Verification items for this drawing (mm, ordinates from the low corner). A direction names the side the tool comes from. Give positions to 0.01 mm unless a question says otherwise; leave off trailing zeros. Loops run counter-clockwise (first coordinate to the right, second up) from the corner with the lowest first, then second, coordinate; pieces in that order, holes last. Notation, with made-up numbers: (-0.5, -25) -> (32.5, -25) arc R17 cw to (32.5, -11) -> close; hole circle Ø5 at (-11, 57). An arc over 180 degrees is marked (long way). Write each question's results on one line, items separated by ' | '. Start each with the question number.
Item 1: Cross-section at B-B on z = 60. Enter the section's corners in (x, y), then the cut area to 3 significant figures.
Item 2: Cross-section at D-D on x = 20. Enter the section's corners in (y, z) (1 decimal).
Item 3: Scan lines: line 1 along Z through (x, y) = (24.5, 15); line 2 along Z through (x, y) = (39, 15); line 3 along Y through (x, z) = (63.5, 15). Record each from-to range of solid material in increasing order.
Item 4: Access from +Z, -Z, +X, -X, +Y, -Y to the whole of each face (thin tool, end or side, straight path). Record for the marked faces 5, 6, 7, 8 and 9.
Item 5: Cross-section at A-A on x = 41. Enter the section's corners in (y, z) (1 decimal).
Item 6: Cross-section at C-C on z = 77. Enter the section's corners in (x, y).
Item 7: Mould release check, pull along Z, two halves, no side actions. Record for the marked faces 1, 2, 3 and 4: pulls with the +Z half, pulls with the -Z half, needs draft (parallel to the pull), parting line crosses it, or undercut.
Item 8: Gauge pin test, flat ends, axial feed: pin 1 Ø15 at (y, z) = (11, 54) entering from -X; pin 2 Ø15 at (y, z) = (15.5, 52.5) entering from +X; pin 3 Ø1 at (x, y) = (15.5, 18) entering from -Z; pin 4 Ø10.5 at (y, z) = (15, 105) entering from -X (1 decimal). Record the tip position at first contact, or that the pin passes through.
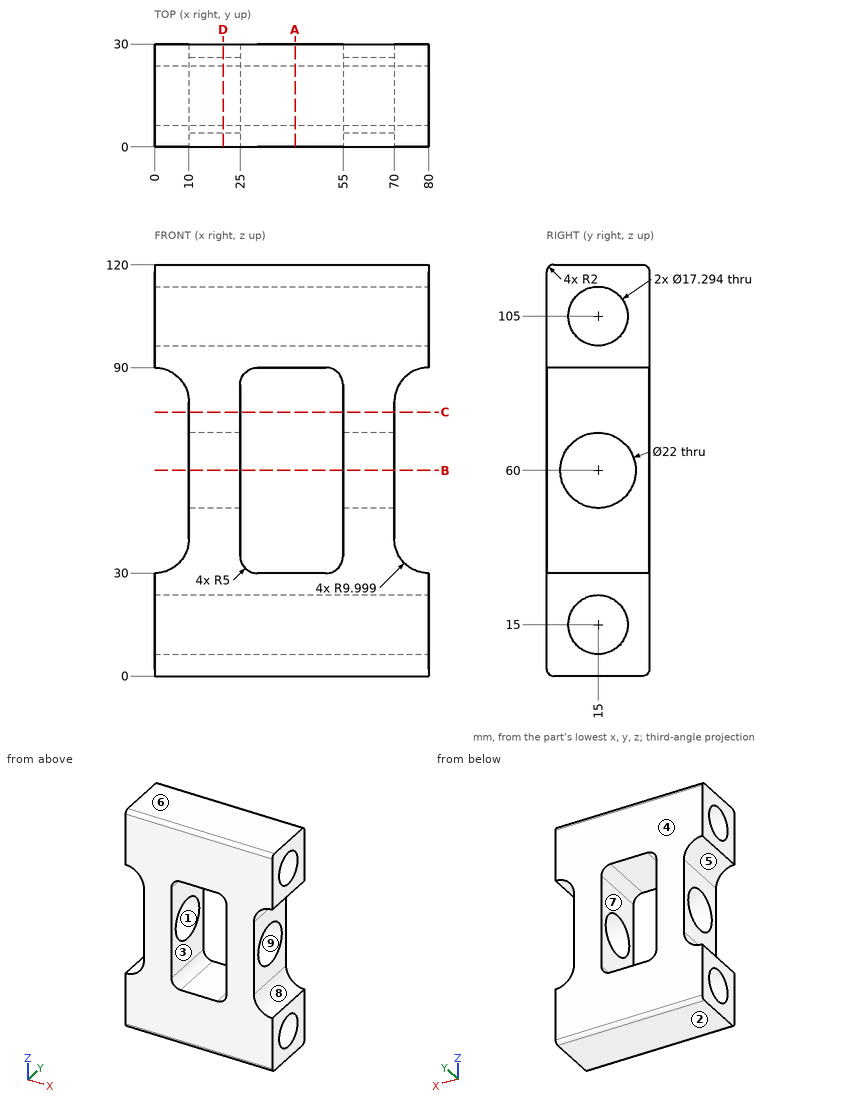
Answer sheet:
1) outline: (10, 0) -> (25, 0) -> (25, 4) -> (10, 4) -> close; (10, 26) -> (25, 26) -> (25, 30) -> (10, 30) -> close; (55, 0) -> (70, 0) -> (70, 4) -> (55, 4) -> close; (55, 26) -> (70, 26) -> (70, 30) -> (55, 30) -> close | area: 240 mm²
2) outline: (0, 2) arc R2 ccw to (2, 0) -> (28, 0) arc R2 ccw to (30, 2) -> (30, 118) arc R2 ccw to (28, 120) -> (2, 120) arc R2 ccw to (0, 118) -> close; hole circle Ø22 at (15, 60); hole circle Ø17.3 at (15, 15); hole circle Ø17.3 at (15, 105)
3) line 1: z = 0 to 6.35, 23.65 to 49, 71 to 96.35, 113.65 to 120 | line 2: z = 0 to 6.35, 23.65 to 30, 90 to 96.35, 113.65 to 120 | line 3: y = 0 to 6.35, 23.65 to 30
4) face 5: -X, +Y, -Y | face 6: +Z, +X, -X, +Y, -Y | face 7: +Y, -Y | face 8: +X, +Y, -Y | face 9: +X, -X
5) outline: (0, 2) arc R2 ccw to (2, 0) -> (28, 0) arc R2 ccw to (30, 2) -> (30, 30) -> (0, 30) -> close; (0, 90) -> (30, 90) -> (30, 118) arc R2 ccw to (28, 120) -> (2, 120) arc R2 ccw to (0, 118) -> close; hole circle Ø17.3 at (15, 15); hole circle Ø17.3 at (15, 105)
6) outline: (10, 0) -> (25, 0) -> (25, 30) -> (10, 30) -> close; (55, 0) -> (70, 0) -> (70, 30) -> (55, 30) -> close
7) face 1: undercut | face 2: pulls with the -Z half | face 3: undercut | face 4: needs draft
8) pin 1: stops at x = 10 | pin 2: stops at x = 70 | pin 3: stops at z = 0 | pin 4: passes through
